from build123d import *

# Parameters (mm, degrees)
BOSS_EXTRUDE1_DEPTH  = 6.35
SKETCH5_W            = 184.15
SKETCH5_H            = 6.35
BOSS_EXTRUDE4_DEPTH  = 31.75
SKETCH6_W            = 12.7
SKETCH6_H            = 88.9
CUT_EXTRUDE2_DEPTH   = 291.872284044
CUT_EXTRUDE3_REACH   = 299.045
SKETCH7_R            = 2.25
SKETCH7_W            = 59.436
SKETCH7_H            = 28.313784743
SKETCH8_R            = 6.35
CUT_EXTRUDE4_DEPTH   = 298.044963979
FILLET1_R            = 2.54
CONVERT_SOLID1_START = -34.925
CONVERT_SOLID1_DEPTH = 184.15
CUT_EXTRUDE5_REACH   = 299.045
CUT_EXTRUDE6_REACH   = 292.872
SKETCH10_R           = 1.63195


# Read off the part's stored shape, not the designer's step: Convert-Solid1
with BuildPart() as part:
    # Sketch1 → Boss-Extrude1 (new body)
    with BuildSketch(Plane(origin=(0, 0, 0), x_dir=(0, 0, -1), z_dir=(1, 0, 0))):
        with BuildLine():
            Line((-117.475, 254), (34.925, 254))
            Line((34.925, 254), (34.925, 8.89))
            Line((34.925, 8.89), (34.925, 0))
            Line((34.925, 0), (-34.925, 0))
            Line((-34.925, 0), (-34.925, 8.89))
            ThreePointArc((-34.925, 8.89), (-79.375, 53.34), (-123.825, 8.89))
            Line((-123.825, 8.89), (-123.825, 0))
            Line((-123.825, 0), (-149.225, 0))
            Line((-149.225, 0), (-149.225, 76.2))
            Line((-149.225, 76.2), (-117.475, 254))
        make_face()
    extrude(amount=BOSS_EXTRUDE1_DEPTH)

    # Sketch5 → Boss-Extrude4 (add)
    with BuildSketch(Plane.ZY):
        with Locations((57.15, 3.175)):
            Rectangle(SKETCH5_W, SKETCH5_H)
    extrude(amount=BOSS_EXTRUDE4_DEPTH)

    # Sketch6 → Cut-Extrude2 (cut, through all)
    with BuildSketch(Plane(origin=(0, 6.35, 0), x_dir=(1, 0, 0), z_dir=(0, 1, 0))):
        with Locations((-6.35, -79.375)):
            Rectangle(SKETCH6_W, SKETCH6_H)
    extrude(amount=-CUT_EXTRUDE2_DEPTH, mode=Mode.SUBTRACT)

    # Sketch7 → Cut-Extrude3 (cut, up to next)
    with BuildSketch(Plane(origin=(6.35, 0, 0), x_dir=(0, 0, -1), z_dir=(1, 0, 0)), mode=Mode.PRIVATE) as cut_extrude3_sk1:
        with Locations((-75.679460058, 116.337237118)):
            Circle(SKETCH7_R)
    cut_extrude3_tool1 = extrude(cut_extrude3_sk1.sketch, amount=-CUT_EXTRUDE3_REACH, mode=Mode.PRIVATE) & part.part
    # Sketch7 → Cut-Extrude3 (cut, up to next)
    with BuildSketch(Plane(origin=(6.35, 0, 0), x_dir=(0, 0, -1), z_dir=(1, 0, 0)), mode=Mode.PRIVATE) as cut_extrude3_sk2:
        with Locations((-75.679460058, 99.360389657)):
            Circle(SKETCH7_R)
    cut_extrude3_tool2 = extrude(cut_extrude3_sk2.sketch, amount=-CUT_EXTRUDE3_REACH, mode=Mode.PRIVATE) & part.part
    # Sketch7 → Cut-Extrude3 (cut, up to next)
    with BuildSketch(Plane(origin=(6.35, 0, 0), x_dir=(0, 0, -1), z_dir=(1, 0, 0)), mode=Mode.PRIVATE) as cut_extrude3_sk3:
        with Locations((-6.03755368, 99.360389657)):
            Circle(SKETCH7_R)
    cut_extrude3_tool3 = extrude(cut_extrude3_sk3.sketch, amount=-CUT_EXTRUDE3_REACH, mode=Mode.PRIVATE) & part.part
    # Sketch7 → Cut-Extrude3 (cut, up to next)
    with BuildSketch(Plane(origin=(6.35, 0, 0), x_dir=(0, 0, -1), z_dir=(1, 0, 0)), mode=Mode.PRIVATE) as cut_extrude3_sk4:
        with Locations((-6.03755368, 116.337237118)):
            Circle(SKETCH7_R)
    cut_extrude3_tool4 = extrude(cut_extrude3_sk4.sketch, amount=-CUT_EXTRUDE3_REACH, mode=Mode.PRIVATE) & part.part
    # Sketch7 → Cut-Extrude3 (cut, up to next)
    with BuildSketch(Plane(origin=(6.35, 0, 0), x_dir=(0, 0, -1), z_dir=(1, 0, 0)), mode=Mode.PRIVATE) as cut_extrude3_sk5:
        with Locations((-40.858506869, 107.848813388)):
            Rectangle(SKETCH7_W, SKETCH7_H)
    cut_extrude3_tool5 = extrude(cut_extrude3_sk5.sketch, amount=-CUT_EXTRUDE3_REACH, mode=Mode.PRIVATE) & part.part
    add(cut_extrude3_tool1.solids().sort_by_distance((6.35, 116.337237, 75.67946))[0], mode=Mode.SUBTRACT)
    add(cut_extrude3_tool2.solids().sort_by_distance((6.35, 99.36039, 75.67946))[0], mode=Mode.SUBTRACT)
    add(cut_extrude3_tool3.solids().sort_by_distance((6.35, 99.36039, 6.037554))[0], mode=Mode.SUBTRACT)
    add(cut_extrude3_tool4.solids().sort_by_distance((6.35, 116.337237, 6.037554))[0], mode=Mode.SUBTRACT)
    add(cut_extrude3_tool5.solids().sort_by_distance((6.35, 107.848813, 40.858507))[0], mode=Mode.SUBTRACT)

    # Sketch8 → Cut-Extrude4 (cut, through all)
    with BuildSketch(Plane(origin=(6.35, 0, 0), x_dir=(0, 0, -1), z_dir=(1, 0, 0))):
        with Locations((-15.875, 209.55)):
            Circle(SKETCH8_R)
    extrude(amount=-CUT_EXTRUDE4_DEPTH, mode=Mode.SUBTRACT)

    # Fillet1
    fillet1_edges = [part.edges().sort_by_distance(p)[0] for p in [
        (0, 6.35, 136.525),
        (0, 6.35, 0),
    ]]
    fillet(fillet1_edges, radius=FILLET1_R)

    # Convert-Solid1 outline → Convert-Solid1 (cut)
    with BuildSketch(Plane.XY.offset(CONVERT_SOLID1_START)):
        with BuildLine():
            ThreePointArc((6.35, 8.89), (3.746179285, 2.603820715), (-2.54, 0))
            Line((-2.54, 0), (6.35, 0))
            Line((6.35, 0), (6.35, 8.89))
        make_face()
    extrude(amount=CONVERT_SOLID1_DEPTH, mode=Mode.SUBTRACT)

    # Sketch9 → Cut-Extrude5 (cut, up to next)
    with BuildSketch(Plane(origin=(6.35, 0, 0), x_dir=(0, 0, -1), z_dir=(1, 0, 0)), mode=Mode.PRIVATE) as cut_extrude5_sk1:
        with BuildLine():
            Line((-75.494212356, 184.752903033), (-73.141435562, 185.731480776))
            ThreePointArc((-73.141435562, 185.731480776), (-69.446832384, 185.812370314), (-66.675, 183.368279277))
            ThreePointArc((-66.675, 183.368279277), (-28.664883279, 153.84953873), (18.415, 163.83))
            ThreePointArc((18.415, 163.83), (27.305, 162.56), (26.035, 153.67))
            ThreePointArc((26.035, 153.67), (-31.616379009, 141.496848075), (-78.066338809, 177.749687467))
            ThreePointArc((-78.066338809, 177.749687467), (-78.311881244, 181.813820193), (-75.494212356, 184.752903033))
        make_face()
    cut_extrude5_tool1 = extrude(cut_extrude5_sk1.sketch, amount=-CUT_EXTRUDE5_REACH, mode=Mode.PRIVATE) & part.part
    add(cut_extrude5_tool1.solids().sort_by_distance((6.35, 181.411079, 77.215324))[0], mode=Mode.SUBTRACT)

    # Sketch10 → Cut-Extrude6 (cut, up to next)
    with BuildSketch(Plane(origin=(0, 6.35, 0), x_dir=(1, 0, 0), z_dir=(0, 1, 0)), mode=Mode.PRIVATE) as cut_extrude6_sk1:
        with Locations(Location((-19.05, 9.525, 0), (0, 0, 270))):
            Circle(SKETCH10_R)
    cut_extrude6_tool1 = extrude(cut_extrude6_sk1.sketch, amount=-CUT_EXTRUDE6_REACH, mode=Mode.PRIVATE) & part.part
    # Sketch10 → Cut-Extrude6 (cut, up to next)
    with BuildSketch(Plane(origin=(0, 6.35, 0), x_dir=(1, 0, 0), z_dir=(0, 1, 0)), mode=Mode.PRIVATE) as cut_extrude6_sk2:
        with Locations(Location((-19.05, -15.875, 0), (0, 0, 270))):
            Circle(SKETCH10_R)
    cut_extrude6_tool2 = extrude(cut_extrude6_sk2.sketch, amount=-CUT_EXTRUDE6_REACH, mode=Mode.PRIVATE) & part.part
    # Sketch10 → Cut-Extrude6 (cut, up to next)
    with BuildSketch(Plane(origin=(0, 6.35, 0), x_dir=(1, 0, 0), z_dir=(0, 1, 0)), mode=Mode.PRIVATE) as cut_extrude6_sk3:
        with Locations(Location((-19.05, -142.875, 0), (0, 0, 270))):
            Circle(SKETCH10_R)
    cut_extrude6_tool3 = extrude(cut_extrude6_sk3.sketch, amount=-CUT_EXTRUDE6_REACH, mode=Mode.PRIVATE) & part.part
    add(cut_extrude6_tool1.solids().sort_by_distance((-19.05, 6.35, -9.525))[0], mode=Mode.SUBTRACT)
    add(cut_extrude6_tool2.solids().sort_by_distance((-19.05, 6.35, 15.875))[0], mode=Mode.SUBTRACT)
    add(cut_extrude6_tool3.solids().sort_by_distance((-19.05, 6.35, 142.875))[0], mode=Mode.SUBTRACT)


solid = part.part
Part model, mm, in its own coordinate system. A direction names the side the tool comes from. Coordinates: 2 decimals unless noted, no trailing zeros. Order: outer loops, then holes, each group sorted by start corner. A loop starts at its lowest first (then second) coordinate and runs counter-clockwise, first axis right, second up.
(1) Slice it at B-B, the plane y = 158.75. Write the cut outline in (x, z) (3 decimals), and give its area (3 significant figures).
Check sheet entries:
outline: (0, -34.925) - (6.35, -34.925) - (6.35, -28.575) - (0, -28.575) - close; (0, -10.307) - (6.35, -10.307) - (6.35, 42.057) - (0, 42.057) - close; (0, 63.816) - (6.35, 63.816) - (6.35, 134.484) - (0, 134.484) - close
area: 822 mm2
(2) Pull direction Z, two halves, no side cores. Call faces 6 (the face through (3, 108, -34.925)), 7 (the face through (-3, 4, 34.925)), 8 (the face through (3, 254, 42)): pulls with the +Z half, pulls with the -Z half, needs draft (parallel to the pull), parting line crosses it, or undercut.
Check sheet entries:
face 6: pulls with the -Z half
face 7: undercut
face 8: needs draft
(3) Pin check, flat tips, straight feed: pin 1 Ø7 at (y, z) = (99.36, 75.68) entering from -X; pin 2 Ø5 at (x, z) = (4, 53.5) entering from -Y; pin 3 Ø10 at (y, z) = (209.55, 15.875) entering from +X; pin 4 Ø3 at (x, y) = (3.5, 105.5) entering from +Z. Stop position of each tip, or through.
Check sheet entries:
pin 1: stops at x = 0
pin 2: stops at y = 43.1
pin 3: passes through
pin 4: stops at z = 144.26
(4) Slice it at A-A, the plane x = -8. Write the cut outline in (y, z) (3 decimals).
Check sheet entries:
outline: (0, -34.925) - (6.35, -34.925) - (6.35, 34.925) - (0, 34.925) - close; (0, 123.825) - (6.35, 123.825) - (6.35, 149.225) - (0, 149.225) - close
(5) Probe L1, parallel to X at y = 244.5, z = 76. List the from-to ranges inside material, lowest first.
Check sheet entries:
L1: x = 0 to 6.35
(6) Tool access for faces 1 (the face through (-12.7, 3, 80)), 2 (the face through (3, 108, 70.577)), 3 (the face through (-31.75, 3, 56)), 4 (the face through (-20, 0, 56)), 5 (the face through (-20, 6.35, 56)): list every direction of +Z, -Z, +X, -X, +Y, -Y with a clear straight run to the whole face (end or side of a thin tool).
Check sheet entries:
face 1: +X, +Y, -Y
face 2: +X, -X
face 3: +Z, -Z, -X, +Y, -Y
face 4: +Z, -Z, +X, -X, -Y
face 5: +Z, -Z, -X, +Y
(7) Slice it at D-D, the plane x = 3.5. State how many separate pieces and enclosed holes the cut face has, and give its area (3 significant figures).
Check sheet entries:
separate pieces: 1
enclosed holes: 7
area: 36,400 mm2
